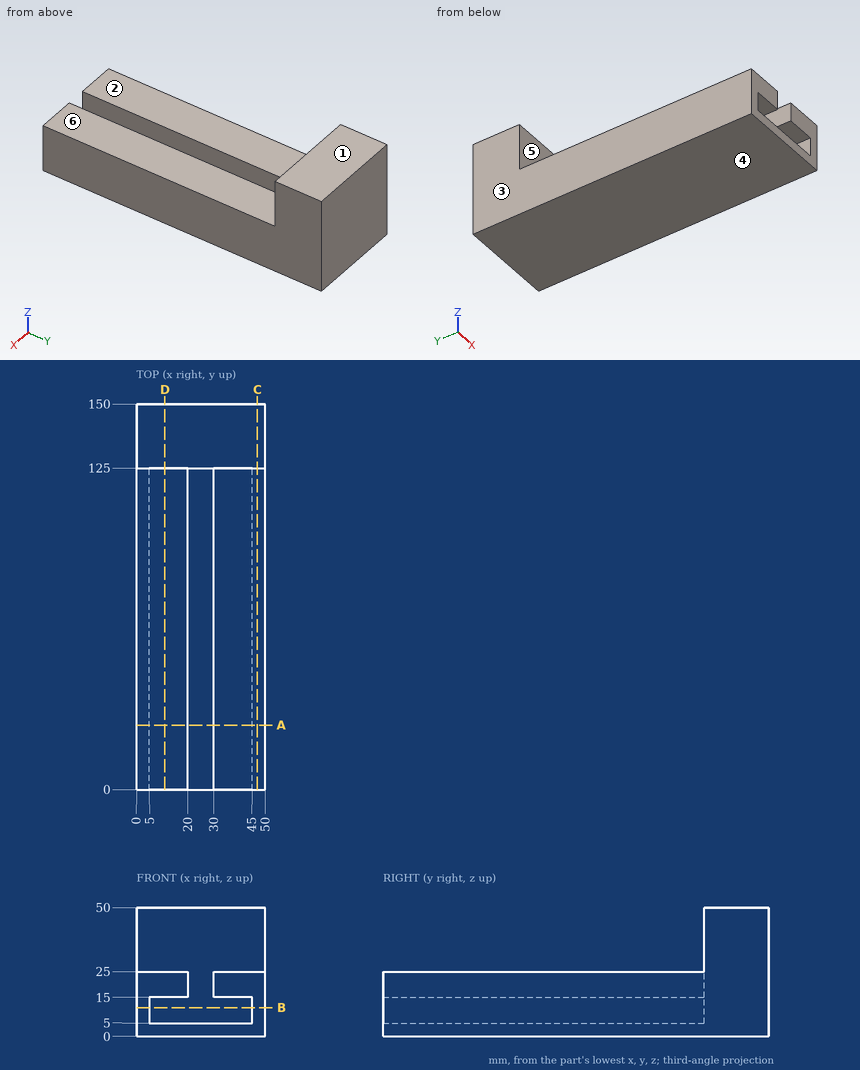
Here's the drawing with two shaded views (mm, measured from the low corner). I have some questions. A direction names the side the tool comes from. Give positions to 0.01 mm unless a question says otherwise; leave off trailing zeros. Loops run counter-clockwise (first coordinate to the right, second up) from the corner with the lowest first, then second, coordinate; pieces in that order, holes last. Notation, with made-up numbers: (62.25, -11) - (119.25, -11) arc R30 ccw to (119.25, 22) - close; hole circle Ø11 at (21.5, -8). An arc over 180 degrees is marked (long way). Return JSON: item names as keys, results as strings.
1. I'm going to push flat-ended pins straight in: pin 1 Ø10 at (x, y) = (11, 49) entering from +Z; pin 2 Ø3 at (x, z) = (38, 7.5) entering from -Y; pin 3 Ø1.5 at (x, y) = (23, 119) entering from +Z. Where does each tip first touch, or does it pass through?
Output values:
{"pin 1": "stops at z = 25", "pin 2": "stops at y = 125", "pin 3": "stops at z = 5"}
2. I want a section at B-B on z = 11. Please give me the cut outline in (x, y), and give its area (3 significant figures).
Output values:
{"outline": "(0, 0) - (5, 0) - (5, 125) - (45, 125) - (45, 0) - (50, 0) - (50, 150) - (0, 150) - close", "area": "2,500 mm²"}
3. For the marked faces 1 and 2, which set-ups out of +Z, -Z, +X, -X, +Y, -Y let a thin tool reach every point of the face, with its end or its side?
Output values:
{"face 1": "+Z, +X, -X, +Y, -Y", "face 2": "+Z, +X, -X, -Y"}
4. I want a section at C-C on x = 47. Please give me the cut outline in (y, z), and give its area (4 significant figures).
Output values:
{"outline": "(0, 0) - (150, 0) - (150, 50) - (125, 50) - (125, 25) - (0, 25) - close", "area": "4,375 mm²"}
5. If I drill on line 1 (Z direction, x = 17.5, y = 31.5); line 2 (X direction, y = 48, z = 7.5); line 3 (Z direction, x = 20.5, y = 54), over which ranges is the centre line in solid material (lowest first)?
Output values:
{"line 1": "z = 0 to 5, 15 to 25", "line 2": "x = 0 to 5, 45 to 50", "line 3": "z = 0 to 5"}
6. I want a section at A-A on y = 25. Please give me the cut outline in (x, z), and give its area (3 significant figures).
Output values:
{"outline": "(0, 0) - (50, 0) - (50, 25) - (30, 25) - (30, 15) - (45, 15) - (45, 5) - (5, 5) - (5, 15) - (20, 15) - (20, 25) - (0, 25) - close", "area": "750 mm²"}
7. We'd pull the mould along Z, two halves only. Please class the marked faces 3, 4, 5 and 6: +Z half, -Z half, draft (parallel to the pull), parting line (faces both ways), or undercut.
Output values:
{"face 3": "draft", "face 4": "-Z half", "face 5": "undercut", "face 6": "+Z half"}
8. I want a section at D-D on x = 11. Please give me the cut outline in (y, z).
Output values:
{"outline": "(0, 0) - (150, 0) - (150, 50) - (125, 50) - (125, 25) - (0, 25) - (0, 15) - (125, 15) - (125, 5) - (0, 5) - close"}
